```python
from build123d import *

# Parameters (mm, degrees)
SKETCH1_R                      = 100
BOSS_EXTRUDE1_DEPTH            = 7.5
CBORE_FOR_M3_SHCS1_D           = 3.4
CBORE_FOR_M3_SHCS1_DEPTH       = 7.5
CBORE_FOR_M3_SHCS1_CBORE_D     = 6.5
CBORE_FOR_M3_SHCS1_CBORE_DEPTH = 3
CBORE_FOR_M3_SHCS1_TIP         = 1.021463052
CBORE_FOR_M3_SHCS2_D           = 3.6
CBORE_FOR_M3_SHCS2_DEPTH       = 7.5
CBORE_FOR_M3_SHCS2_CBORE_D     = 6.5
CBORE_FOR_M3_SHCS2_CBORE_DEPTH = 3
CBORE_FOR_M3_SHCS2_TIP         = 1.081549114
SKETCH9_W                      = 276.839915284
SKETCH9_H                      = 86.454597136
CUT_EXTRUDE1_DEPTH             = 142.620090383
SKETCH11_R                     = 1.875
BOSS_EXTRUDE3_DEPTH            = 1.875
FILLET1_R                      = 1.875


with BuildPart() as part:
    # Sketch1 → Boss-Extrude1 (new body)
    with BuildSketch(Plane(origin=(0, 0, 0), x_dir=(1, 0, 0), z_dir=(0, 1, 0))):
        with Locations(Location((0, 0, 0), (0, 0, 270))):
            Circle(SKETCH1_R)
    extrude(amount=BOSS_EXTRUDE1_DEPTH)

    # CBORE for M3 SHCS1
    with Locations(Plane(origin=(0, 0, 0), x_dir=(-1, 0, 0), z_dir=(0, -1, 0))):
        with Locations((0, -92.5), (-65.40737726, -65.40737726), (-92.5, 0), (-65.40737726, 65.40737726), (0, 92.5), (65.40737726, 65.40737726), (92.5, 0), (65.40737726, -65.40737726)):
            CounterBoreHole(CBORE_FOR_M3_SHCS1_D / 2, CBORE_FOR_M3_SHCS1_CBORE_D / 2, CBORE_FOR_M3_SHCS1_CBORE_DEPTH, depth=CBORE_FOR_M3_SHCS1_DEPTH)
            with Locations((0, 0, -(CBORE_FOR_M3_SHCS1_DEPTH + CBORE_FOR_M3_SHCS1_TIP / 2))):  # 118° drill point
                Cone(0, CBORE_FOR_M3_SHCS1_D / 2, CBORE_FOR_M3_SHCS1_TIP, mode=Mode.SUBTRACT)

    # CBORE for M3 SHCS2
    with Locations(Plane(origin=(0, 0, 0), x_dir=(-1, 0, 0), z_dir=(0, -1, 0))):
        with Locations((-53, 34), (53, 34), (53, -34), (-53, -34)):
            CounterBoreHole(CBORE_FOR_M3_SHCS2_D / 2, CBORE_FOR_M3_SHCS2_CBORE_D / 2, CBORE_FOR_M3_SHCS2_CBORE_DEPTH, depth=CBORE_FOR_M3_SHCS2_DEPTH)
            with Locations((0, 0, -(CBORE_FOR_M3_SHCS2_DEPTH + CBORE_FOR_M3_SHCS2_TIP / 2))):  # 118° drill point
                Cone(0, CBORE_FOR_M3_SHCS2_D / 2, CBORE_FOR_M3_SHCS2_TIP, mode=Mode.SUBTRACT)

    # Sketch9 → Cut-Extrude1 (cut, through all)
    with BuildSketch(Plane(origin=(0, 0, 0), x_dir=(0.3646980843717534, 0, 0.9311258278318637), z_dir=(-0.9311258278318637, 0, 0.3646980843717534))):
        with Locations((-1.022117504, -7.168579764)):
            Rectangle(SKETCH9_W, SKETCH9_H)
    extrude(amount=CUT_EXTRUDE1_DEPTH, mode=Mode.SUBTRACT)

    # Sketch11 → Boss-Extrude3 (add)
    with BuildSketch(Plane(origin=(0, 0, 0), x_dir=(0.3646980843717534, 0, 0.9311258278318637), z_dir=(-0.9311258278318637, 0, 0.3646980843717534))):
        with Locations(Location((0, 3.75, 0), (0, 0, 180))):
            Circle(SKETCH11_R)
        with Locations(Location((-40, 3.75, 0), (0, 0, 180))):
            Circle(SKETCH11_R)
        with Locations(Location((-80, 3.75, 0), (0, 0, 180))):
            Circle(SKETCH11_R)
        with Locations(Location((80, 3.75, 0), (0, 0, 180))):
            Circle(SKETCH11_R)
        with Locations(Location((40, 3.75, 0), (0, 0, 180))):
            Circle(SKETCH11_R)
    extrude(amount=BOSS_EXTRUDE3_DEPTH)

    # Fillet1
    fillet1_edges = [part.edges().sort_by_distance(p)[0] for p in [
        (-1.062052019, 3.75, 2.429669835),
        (-15.649975394, 3.75, -34.815363278),
        (-30.237898769, 3.75, -72.060396391),
        (28.113794731, 3.75, 76.919736062),
        (13.525871356, 3.75, 39.674702949),
    ]]
    fillet(fillet1_edges, radius=FILLET1_R - 0.0001)  # a hair under: the kernel refuses the full size


solid = part.part
```
Verification items for the finished model (mm, model axes). A direction names the side the tool comes from. Coordinates: 2 decimals unless noted, no trailing zeros. Write each loop counter-clockwise with the first axis right and the second up, starting at its lowest first coordinate (ties: lowest second). Pieces come first, ordered by that corner, then holes. Notation, with made-up numbers: M 38.25,55 L 82.25,55 A33 cw 82.25,83 Z; hole C 18,49 d2. An arc over 180 degrees is marked long. Answer as a JSON object with one key per item and string values. Group by question number.
(1) Material ranges on line 1 (Z direction, x = 53, y = 5.7); line 2 (Z direction, x = 56, y = 2.75), recorded low to high.
(2) Cross-section at A-A, the plane x = 74.5. Record the cut outline in (y, z), and give its area (3 significant figures).
(3) Release check for a two-part mould opening along Z. For faces 3 (the face through (33, 7.5, -5)), 4 (the face through (91.1, 3, 1.4)), 5 (the face through (93.892, 3.698, -34.414)) record: +Z half, -Z half, draft (parallel to the pull), parting line (faces both ways), or undercut.
(4) Cross-section at B-B, the plane z = -87. Record the cut outline in (x, y).
(5) Tool access check on faces 1 (the face through (52.766, 5.281, -35.785)), 2 (the face through (64, 3, -64)). Record the directions out of +Z, -Z, +X, -X, +Y, -Y that give a thin tool (end or side, any length) a straight path to the whole face; none if there is none.
(6) Gauge pin test, flat ends, axial feed: pin 1 (5 mm diameter, centred on x = 0, z = -92, fed in from -Y); pin 2 (1 mm diameter, centred on x = 78, y = 1.5, fed in from +Z). Record the tip position at first contact, or that the pin passes through.
Reply:
{
 "1": {"line 1": "-84.8 to -35.8, -32.2 to 32.2, 35.8 to 84.8", "line 2": "-82.85 to -35.25, -32.75 to 32.75, 35.25 to 82.85"},
 "2": {"outline": "M 0,-66.71 L 7.5,-66.71 L 7.5,66.71 L 0,66.71 Z", "area": "1,000 mm²"},
 "3": {"face 3": "draft", "face 4": "undercut", "face 5": "parting line"},
 "4": {"outline": "M -34.08,0 L 49.31,0 L 49.31,7.5 L -34.08,7.5 Z"},
 "5": {"face 1": "+Y, -Y", "face 2": "-Y"},
 "6": {"pin 1": "y = 3", "pin 2": "z = 63.2"}
}
